Design review of the part shown in the three views and the two pictorial views. Dimensions are in mm from the part's minimum x, y and z. A direction names the side the tool comes from. Give positions to 0.01 mm unless a question says otherwise; leave off trailing zeros. Loops run counter-clockwise (first coordinate to the right, second up) from the corner with the lowest first, then second, coordinate; pieces in that order, holes last. Notation, with made-up numbers: M -17.5,84.5 L 13.5,84.5 A15 cw 13.5,94.5 Z; hole C 33.25,8.25 d3. An arc over 180 degrees is marked long. Return JSON: item names as keys, results as strings. Group by question number.
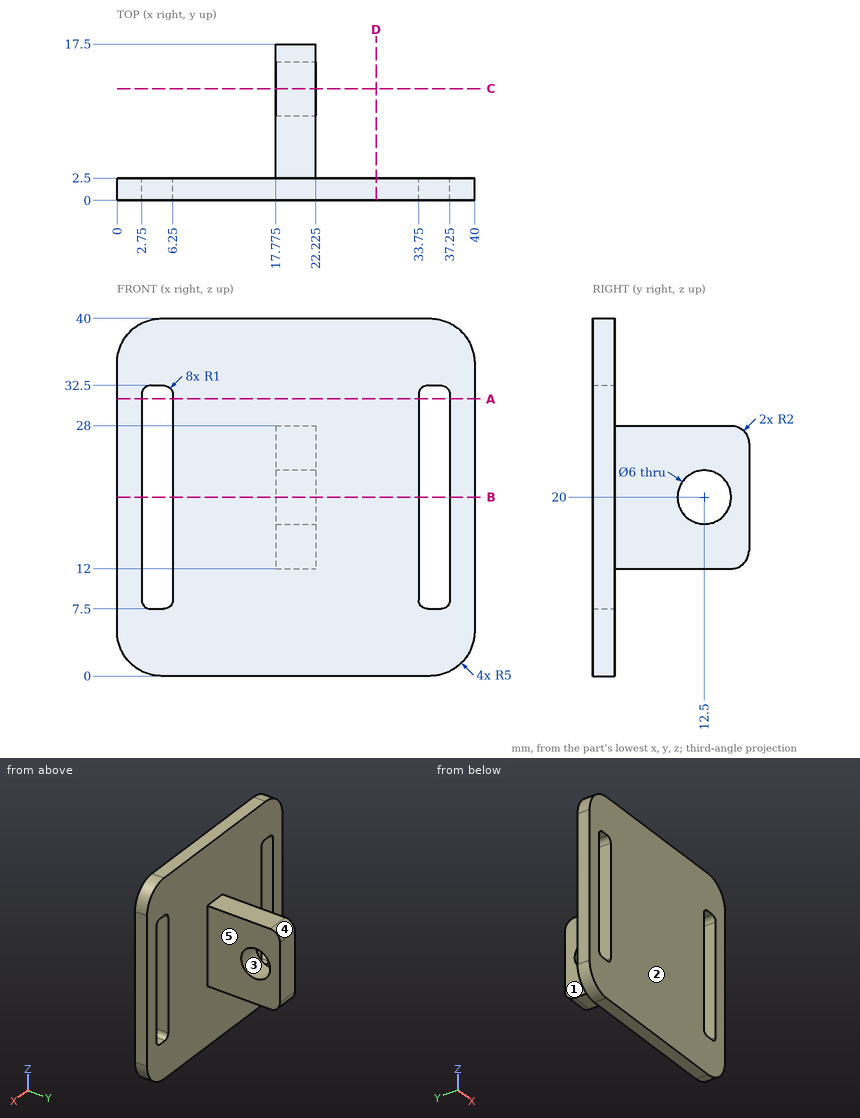
(1) For pin 1 (5 mm diameter, centred on x = 23, y = 8, fed in from -Z); pin 2 (4 mm diameter, centred on x = 28.5, z = 32.5, fed in from +Y); pin 3 (4.5 mm diameter, centred on y = 10.5, z = 22, fed in from +X) (3 decimals); pin 4 (3.5 mm diameter, centred on y = 12.5, z = 20, fed in from +X), all flat-tipped, find the tip position at first contact; note any pin that passes through.
(2) Add section D-D (x = 29). Write out the cut boundary in (y, z), and give its area (3 significant figures).
(3) For the marked faces 1 and 2, list the 3-axis set-ups (+Z, -Z, +X, -X, +Y, -Y) from which the entire face can be reached by the end or side of a thin tool; tool diameter is ignored.
(4) Add section B-B (z = 20). Write out the cut boundary in (x, y) (3 decimals).
(5) Mouldability with a two-part tool opening along Z and no side actions: class the marked faces 3, 4 and 5 as released by +Z, released by -Z, zero draft, split by the parting line, or undercut.
(6) For probe 1 along Y at (x, z) = (20, 20); probe 2 along Z at (x, y) = (19.2, 12.5); probe 3 along Y at (x, z) = (26, 4), list the stretches that pass through material, from the lowest coordinate up.
(7) Add section A-A (z = 31). Write out the cut boundary in (x, y).
(8) Add section C-C (y = 12.5). Write out the cut boundary in (x, z) (3 decimals).
Verdict:
{
 "1": {"pin 1": "stops at z = 12", "pin 2": "stops at y = 2.5", "pin 3": "stops at x = 22.225", "pin 4": "passes through"},
 "2": {"outline": "M 0,0 L 2.5,0 L 2.5,40 L 0,40 Z", "area": "100 mm²"},
 "3": {"face 1": "+Z, -Z, -X, +Y", "face 2": "+Z, -Z, +X, -X, -Y"},
 "4": {"outline": "M 0,0 L 2.75,0 L 2.75,2.5 L 0,2.5 Z; M 6.25,0 L 33.75,0 L 33.75,2.5 L 22.225,2.5 L 22.225,9.5 L 17.775,9.5 L 17.775,2.5 L 6.25,2.5 Z; M 17.775,15.5 L 22.225,15.5 L 22.225,17.5 L 17.775,17.5 Z; M 37.25,0 L 40,0 L 40,2.5 L 37.25,2.5 Z"},
 "5": {"face 3": "undercut", "face 4": "released by +Z", "face 5": "zero draft"},
 "6": {"probe 1": "y = 0 to 9.5, 15.5 to 17.5", "probe 2": "z = 12 to 17, 23 to 28", "probe 3": "y = 0 to 2.5"},
 "7": {"outline": "M 0,0 L 2.75,0 L 2.75,2.5 L 0,2.5 Z; M 6.25,0 L 33.75,0 L 33.75,2.5 L 6.25,2.5 Z; M 37.25,0 L 40,0 L 40,2.5 L 37.25,2.5 Z"},
 "8": {"outline": "M 17.775,12 L 22.225,12 L 22.225,17 L 17.775,17 Z; M 17.775,23 L 22.225,23 L 22.225,28 L 17.775,28 Z"}
}
